Geometry check sheet. Reference: the model listing, model coordinates, mm. A direction names the side the tool comes from. Give positions to 0.01 mm unless a question says otherwise; leave off trailing zeros. Order: outer loops, then holes, each group sorted by start corner. A loop starts at its lowest first (then second) coordinate and runs counter-clockwise, first axis right, second up. Notation, with made-up numbers: M 38,32 L 88,32 A18 ccw 88,65 Z; hole C 38,-11 d11. An arc over 180 degrees is marked long. Answer as CSV lines item,"result". Start each with the question number.
Q1. Section check A-A, the plane z = -12.5. Count the separate pieces of the cut face and the enclosed holes in it, then the cut area to 3 significant figures.
Q2. Go/stop test with flat-tipped pins: pin 1 (1.6 mm diameter, centred on y = 30.5, z = -12.5, fed in from +X); pin 2 (1.5 mm diameter, centred on x = 44.5, z = -24.5, fed in from +Y); pin 3 (5.5 mm diameter, centred on y = 42, z = -23, fed in from -X). Record where each tip stops, or that it passes through.
Q3. Section check C-C, the plane y = 9. Record the boundary of the cut face in (x, z) (3 decimals), then the cut area to 3 significant figures.
Q4. Thickness scan on line 1 (Y direction, x = 53.5, z = -12.5); line 2 (Y direction, x = 50, z = -14.5); line 3 (Z direction, x = 4, y = 40) (3 decimals). Record the ranges inside material, lowest first.
Q5. Section check B-B, the plane x = 4. Record the boundary of the cut face in (y, z) (3 decimals).
Q6. Section check D-D, the plane y = 19. Record the boundary of the cut face in (x, z), then the cut area to 3 significant figures.
Q7. Mould release check, pull along X, two halves, no side actions. Record for faces 1 (the flat face through (5.5, 41, -2)), 2 (the cylindrical face through (-4.5, 7.2, -12.4)), 3 (the cylindrical face through (51.556, 29.545, -12.28)): +X half, -X half, draft (parallel to the pull), parting line (faces both ways), or undercut.
Q8. Set-up check for faces 4 (the flat face through (47.5, 3, -13)), 5 (the flat face through (4, 37, -20)), 6 (the flat face through (8, 14.167, -13)), 7 (the flat face through (0, 41, -27)): record each of +Z, -Z, +X, -X, +Y, -Y from which the full face is reachable in a straight line by a thin tool's end or side.
```python
from build123d import *

# Parameters (mm, degrees)
BOSS_EXTRUDE1_DEPTH = 55.5
CHAMFER1_SIZE       = 2
SKETCH4_W           = 8
SKETCH4_H           = 32.8
BOSS_EXTRUDE2_DEPTH = 5
SKETCH7_W           = 3.5
SKETCH7_H           = 6
CUT_EXTRUDE5_DEPTH  = 10
SKETCH5_R           = 3.375
CUT_EXTRUDE3_DEPTH  = 77.250596562
SKETCH6_R           = 3.375
CUT_EXTRUDE4_DEPTH  = 7.62
SKETCH8_W           = 9
SKETCH8_H           = 5
CUT_EXTRUDE6_DEPTH  = 9.167
BOSS_EXTRUDE3_DEPTH = 14.167
BOSS_EXTRUDE4_START = -29.407
BOSS_EXTRUDE4_DEPTH = 14.167
FILLET1_R           = 10
SKETCH10_W          = 15
SKETCH10_H          = 25
CUT_EXTRUDE7_DEPTH  = 20
SKETCH11_R          = 1.016
CUT_EXTRUDE8_DEPTH  = 8
SKETCH12_W          = 5
SKETCH12_H          = 12
CUT_EXTRUDE9_DEPTH  = 14.437


with BuildPart() as part:
    # Sketch1 → Boss-Extrude1 (new body)
    with BuildSketch(Plane(origin=(0, 0, 0), x_dir=(0, 0, -1), z_dir=(1, 0, 0))):
        Polygon((0, 0), (25, 0), (25, 19.787), (21.5, 21.787), (25, 23.787), (25, 43.574), (0, 43.574), (0, 23.787), (3.5, 21.787), (0, 19.787), align=None)
    extrude(amount=BOSS_EXTRUDE1_DEPTH)

    # Chamfer1
    chamfer1_edges = [part.edges().sort_by_distance(p)[0] for p in [
        (27.75, 43.574, 0),
        (27.75, 43.574, -25),
        (27.75, 0, -25),
        (27.75, 0, 0),
    ]]
    chamfer(chamfer1_edges, length=CHAMFER1_SIZE)

    # Sketch4 → Boss-Extrude2 (add)
    with BuildSketch(Plane(origin=(0, 43.574, 0), x_dir=(1, 0, 0), z_dir=(0, 1, 0))):
        with Locations((4, 12.5)):
            Rectangle(SKETCH4_W, SKETCH4_H)
    extrude(amount=-BOSS_EXTRUDE2_DEPTH)

    # Sketch7 → Cut-Extrude5 (cut)
    with BuildSketch(Plane(origin=(0, 43.574, 0), x_dir=(1, 0, 0), z_dir=(0, 1, 0))):
        with Locations((7.25, 2)):
            Rectangle(SKETCH7_W, SKETCH7_H)
        with Locations((7.25, 23)):
            Rectangle(SKETCH7_W, SKETCH7_H)
        with Locations((0.75, 2)):
            Rectangle(SKETCH7_W, SKETCH7_H)
        with Locations((0.75, 23)):
            Rectangle(SKETCH7_W, SKETCH7_H)
    extrude(amount=-CUT_EXTRUDE5_DEPTH, mode=Mode.SUBTRACT)

    # Sketch5 → Cut-Extrude3 (cut, through all)
    with BuildSketch(Plane(origin=(0, 43.574, 0), x_dir=(1, 0, 0), z_dir=(0, 1, 0))):
        with Locations(Location((4, 12.5, 0), (0, 0, 270))):
            Circle(SKETCH5_R)
    extrude(amount=-CUT_EXTRUDE3_DEPTH, mode=Mode.SUBTRACT)

    # Sketch6 → Cut-Extrude4 (cut, symmetric)
    with BuildSketch(Plane(origin=(0, 21.787, 0), x_dir=(-1, 0, 0), z_dir=(0, -1, 0))):
        Polygon((-4, 30), (4.5, 30), (4.5, -5), (-4, -5), (-15.5, -5), (-15.5, 30), align=None)
        with Locations(Location((-4, 12.5, 0), (0, 0, 270))):
            Circle(SKETCH6_R, mode=Mode.SUBTRACT)
    extrude(amount=CUT_EXTRUDE4_DEPTH, both=True, mode=Mode.SUBTRACT)

    # Sketch8 → Cut-Extrude6 (cut)
    with BuildSketch(Plane.XZ.offset(-29.407)):
        with Locations((4.5, -22.5)):
            Rectangle(SKETCH8_W, SKETCH8_H)
        with Locations((4.5, -2.5)):
            Rectangle(SKETCH8_W, SKETCH8_H)
    extrude(amount=-CUT_EXTRUDE6_DEPTH, mode=Mode.SUBTRACT)

    # Sketch9 → Boss-Extrude3 (add)
    with BuildSketch(Plane(origin=(0, 43.574, 0), x_dir=(1, 0, 0), z_dir=(0, 1, 0))):
        with BuildLine():
            Line((0, 20), (0, 5))
            ThreePointArc((0, 5), (-4.5, 12.5), (0, 20))
        make_face()
    extrude(amount=-BOSS_EXTRUDE3_DEPTH)

    # Sketch9<2> → Boss-Extrude4 (add)
    with BuildSketch(Plane(origin=(0, 43.574, 0), x_dir=(1, 0, 0), z_dir=(0, 1, 0)).offset(BOSS_EXTRUDE4_START)):
        with BuildLine():
            Line((0, 20), (0, 5))
            ThreePointArc((0, 5), (-4.5, 12.5), (0, 20))
        make_face()
    extrude(amount=-BOSS_EXTRUDE4_DEPTH)

    # Fillet1
    fillet1_edges = [part.edges().sort_by_distance(p)[0] for p in [
        (0, 7.0835, -20),
        (0, 7.0835, -5),
    ]]
    fillet(fillet1_edges, radius=FILLET1_R)

    # Sketch10 → Cut-Extrude7 (cut)
    with BuildSketch(Plane(origin=(55.5, 0, 0), x_dir=(0, 0, -1), z_dir=(1, 0, 0))):
        with Locations((12.5, 16.637)):
            Rectangle(SKETCH10_W, SKETCH10_H)
    extrude(amount=-CUT_EXTRUDE7_DEPTH, mode=Mode.SUBTRACT)

    # Sketch11 → Cut-Extrude8 (cut)
    with BuildSketch(Plane(origin=(55.5, 0, 0), x_dir=(0, 0, -1), z_dir=(1, 0, 0))):
        with Locations((12.5, 30.537)):
            Circle(SKETCH11_R)
        with Locations(Location((12.5, 2.737, 0), (0, 0, 180))):
            Circle(SKETCH11_R)
    extrude(amount=-CUT_EXTRUDE8_DEPTH, mode=Mode.SUBTRACT)

    # Sketch12 → Cut-Extrude9 (cut)
    with BuildSketch(Plane(origin=(0, 43.574, 0), x_dir=(1, 0, 0), z_dir=(0, 1, 0))):
        with Locations((38, 12.5)):
            Rectangle(SKETCH12_W, SKETCH12_H)
    extrude(amount=-CUT_EXTRUDE9_DEPTH, mode=Mode.SUBTRACT)


solid = part.part
```
Answer block:
1,separate pieces,"4"
1,enclosed holes,"0"
1,area,"1,510 mm2"
2,pin 1,"stops at x = 47.5"
2,pin 2,"stops at y = 42.82"
2,pin 3,"stops at x = 2.5"
3,outline,"M -2.432,-18.056 A10 cw 0,-24.593 L 0,-25 L 55.5,-25 L 55.5,-20 L 35.5,-20 L 35.5,-5 L 55.5,-5 L 55.5,0 L 0,0 L 0,-0.407 A10 cw -2.432,-6.944 A8.5 ccw Z; hole C 4,-12.5 d6.75"
3,area,"1,100 mm2"
4,line 1,"y = 0 to 1.72, 3.75 to 4.14, 29.14 to 29.52, 31.55 to 43.57"
4,line 2,"y = 0 to 4.14, 29.14 to 43.57"
4,line 3,"z = -28.9 to -15.875, -9.125 to 3.9"
5,outline,"M 0,-23 L 2,-25 L 14.167,-25 L 14.167,-15.875 L 0,-15.875 Z; M 0,-9.125 L 14.167,-9.125 L 14.167,0 L 2,0 L 0,-2 Z; M 29.407,-20 L 38.574,-20 L 38.574,-28.9 L 43.574,-28.9 L 43.574,-15.875 L 29.407,-15.875 Z; M 29.407,-9.125 L 43.574,-9.125 L 43.574,3.9 L 38.574,3.9 L 38.574,-5 L 29.407,-5 Z"
6,outline,"M 15.5,-25 L 55.5,-25 L 55.5,-20 L 35.5,-20 L 35.5,-5 L 55.5,-5 L 55.5,0 L 15.5,0 Z"
6,area,"700 mm2"
7,face 1,"undercut"
7,face 2,"-X half"
7,face 3,"draft"
8,face 4,"+X"
8,face 5,"none"
8,face 6,"+Z, -Z, -X"
8,face 7,"-Z, -X, +Y, -Y"
